Verification items for the finished model (mm, model axes). Round coordinates to 2 decimals unless told otherwise and drop trailing zeros. Write each loop counter-clockwise with the first axis right and the second up, starting at its lowest first coordinate (ties: lowest second). Pieces come first, ordered by that corner, then holes. Notation, with made-up numbers: M 32.25,-4 L 73.25,-4 A20 ccw 73.25,25 Z; hole C 10.25,34 d2. An arc over 180 degrees is marked long. One line per item, written item: value. Start each with the question number.
from build123d import *

# Parameters (mm, degrees)
SKETCH3_R           = 74.295
SKETCH3_R_2         = 3.175
SKETCH3_R_3         = 5.842
BOSS_EXTRUDE2_DEPTH = 3.175
CUT_EXTRUDE2_DEPTH  = 4.175


with BuildPart() as part:
    # Sketch3 → Boss-Extrude2 (new body)
    with BuildSketch(Plane.XY):
        Circle(SKETCH3_R)
        with Locations((-32.198217622, 56.128319663)):
            Circle(SKETCH3_R_2, mode=Mode.SUBTRACT)
        with Locations((32.322739207, 56.128319663)):
            Circle(SKETCH3_R_2, mode=Mode.SUBTRACT)
        with Locations((-32.322739207, -56.128319663)):
            Circle(SKETCH3_R_2, mode=Mode.SUBTRACT)
        with Locations((32.198217622, -56.128319663)):
            Circle(SKETCH3_R_2, mode=Mode.SUBTRACT)
        Circle(SKETCH3_R_3, mode=Mode.SUBTRACT)
    extrude(amount=BOSS_EXTRUDE2_DEPTH)

    # Sketch4 → Cut-Extrude2 (cut, through all)
    with BuildSketch(Plane.XY.offset(3.175)):
        with BuildLine():
            Line((-48.930202294, 55.906907699), (-48.930202294, -55.906907699))
            ThreePointArc((-48.930202294, -55.906907699), (-74.295, 0), (-48.930202294, 55.906907699))
        make_face()
        with BuildLine():
            Line((48.930202294, 55.906907699), (48.930202294, -55.906907699))
            ThreePointArc((48.930202294, -55.906907699), (74.295, 0), (48.930202294, 55.906907699))
        make_face()
    extrude(amount=-CUT_EXTRUDE2_DEPTH, mode=Mode.SUBTRACT)


solid = part.part
1) Mould release check, pull along X, two halves, no side actions. Record for faces 1 (the cylindrical face through (0.75, 74.29, 1.57)), 2 (the cylindrical face through (-30.62, -53.45, 1.57)), 3 (the cylindrical face through (29.98, 58.27, 1.57)), 4 (the flat face through (48.93, 1, 2)): pulls with the +X half, pulls with the -X half, needs draft (parallel to the pull), parting line crosses it, or undercut.
2) Cross-section at D-D (y = 63.5). Record the boundary of the cut face in (x, z) (3 decimals).
3) Cross-section at C-C (z = 1.05). Record the boundary of the cut face in (x, y) (3 decimals).
4) Thickness scan on line 1 (X direction, y = -3.5, z = 0.55); line 2 (Y direction, x = 33, z = 1.65); line 3 (X direction, y = 56.5, z = 1.65). Record the ranges inside material, lowest first.
5) Cross-section at A-A (y = 0). Record the boundary of the cut face in (x, z) (3 decimals).
6) Cross-section at B-B (x = 0). Record the boundary of the cut face in (y, z) (3 decimals), then the cut area to 3 significant figures.
Results below:
1. face 1: parting line crosses it
1. face 2: undercut
1. face 3: undercut
1. face 4: pulls with the +X half
2. outline: M -38.568,0 L 38.568,0 L 38.568,3.175 L -38.568,3.175 Z
3. outline: M -48.93,-55.907 A74.295 ccw 48.93,-55.907 L 48.93,55.907 A74.295 ccw -48.93,55.907 Z; hole C -32.323,-56.128 d6.35; hole C -32.198,56.128 d6.35; hole C 0,0 d11.684; hole C 32.198,-56.128 d6.35; hole C 32.323,56.128 d6.35
4. line 1: x = -48.93 to -4.68, 4.68 to 48.93
4. line 2: y = -66.56 to -59.2, -53.06 to 53.03, 59.23 to 66.56
4. line 3: x = -48.24 to -35.35, -29.05 to 29.17, 35.48 to 48.24
5. outline: M -48.93,0 L -5.842,0 L -5.842,3.175 L -48.93,3.175 Z; M 5.842,0 L 48.93,0 L 48.93,3.175 L 5.842,3.175 Z
6. outline: M -74.295,0 L -5.842,0 L -5.842,3.175 L -74.295,3.175 Z; M 5.842,0 L 74.295,0 L 74.295,3.175 L 5.842,3.175 Z
6. area: 435 mm²
